Design review of the part built by this model. Coordinates are the model's own, in mm. A direction names the side the tool comes from. Give positions to 0.01 mm unless a question says otherwise; leave off trailing zeros. Loops run counter-clockwise (first coordinate to the right, second up) from the corner with the lowest first, then second, coordinate; pieces in that order, holes last. Notation, with made-up numbers: M 82.25,-33.75 L 111.25,-33.75 A16 ccw 111.25,-25.75 Z; hole C 23.5,44 d3. An arc over 180 degrees is marked long. Answer as CSV lines item,"result".
```python
from build123d import *

# Parameters (mm, degrees)
ESQUISSE1_W        = 5
ESQUISSE1_H        = 7
BOSS_EXTRU_1_DEPTH = 2.5
ESQUISSE2_R        = 0.25
BOSS_EXTRU_2_DEPTH = 23
ESQUISSE3_W        = 4
ESQUISSE3_H        = 6
BOSS_EXTRU_3_DEPTH = 2
CONG_1_R           = 2


with BuildPart() as part:
    # Esquisse1 → Boss.-Extru.1 (new body)
    with BuildSketch(Plane(origin=(0, 0, 0), x_dir=(1, 0, 0), z_dir=(0, 1, 0))):
        with Locations((2.5, 3.5)):
            Rectangle(ESQUISSE1_W, ESQUISSE1_H)
    extrude(amount=BOSS_EXTRU_1_DEPTH)

    # Esquisse2 → Boss.-Extru.2 (add)
    with BuildSketch(Plane.XY):
        with Locations(Location((0.5, 1.25, 0), (0, 0, 180))):
            Circle(ESQUISSE2_R)
        with Locations(Location((2.5, 1.25, 0), (0, 0, 180))):
            Circle(ESQUISSE2_R)
        with Locations(Location((4.5, 1.25, 0), (0, 0, 180))):
            Circle(ESQUISSE2_R)
    extrude(amount=BOSS_EXTRU_2_DEPTH)

    # Esquisse3 → Boss.-Extru.3 (add)
    with BuildSketch(Plane(origin=(0, 2.5, 0), x_dir=(1, 0, 0), z_dir=(0, 1, 0))):
        with Locations((2.5, 3)):
            Rectangle(ESQUISSE3_W, ESQUISSE3_H)
    extrude(amount=BOSS_EXTRU_3_DEPTH)

    # Congé1
    cong_1_edges = [part.edges().sort_by_distance(p)[0] for p in [
        (4.5, 4.5, -3),
        (2.5, 4.5, -6),
        (0.5, 4.5, -3),
    ]]
    fillet(cong_1_edges, radius=CONG_1_R - 0.0001)  # a hair under: the kernel refuses the full size


solid = part.part
```
1. For P1, Ø3, axis at x = 4.5, z = 10.5, coming from the -Y side; P2, Ø3, axis at x = 1, z = 13, coming from the +Y side, all flat-tipped, find the tip position at first contact; note any pin that passes through.
Answer block:
P1,"y = 1"
P2,"y = 1.5"
2. For faces 1 (the flat face through (2.3, 2.5, -6.4)), 2 (the flat face through (2, 0, -4)), list the 3-axis set-ups (+Z, -Z, +X, -X, +Y, -Y) from which the entire face can be reached by the end or side of a thin tool; tool diameter is ignored.
Answer block:
face 1,"-Z, +Y"
face 2,"+Z, -Z, +X, -X, -Y"
3. We need section B-B, the plane z = 14. Write out the cut boundary in (x, y).
Answer block:
outline,"C 0.5,1.25 d0.5; C 2.5,1.25 d0.5; C 4.5,1.25 d0.5"
4. We need section D-D, the plane y = 4.2. Write out the cut boundary in (x, z).
Answer block:
outline,"M 1.45,-5.05 L 3.55,-5.05 L 3.55,0 L 1.45,0 Z"
5. To check wall thickness, follow L1, parallel to X at y = 1.2, z = 10.75; L2, parallel to Z at x = 3, y = 2.15; L3, parallel to Z at x = 4.2, y = 2.6. State the ranges of each line that lie inside material, in increasing order. Write a range as [from, to].
Answer block:
L1,"[0.26, 0.74], [2.26, 2.74], [4.26, 4.74]"
L2,"[-7, 0]"
L3,"[-6, 0]"
6. The part is to be moulded in two halves that separate along Z. For faces 3 (the cylindrical face through (2.53, 3.63, -5.65)), 4 (the flat face through (2, 2, 0)), 5 (the flat face through (0, 1, -3)), say which applies: pulls with the +Z half, pulls with the -Z half, needs draft (parallel to the pull), parting line crosses it, or undercut.
Answer block:
face 3,"pulls with the -Z half"
face 4,"pulls with the +Z half"
face 5,"needs draft"
7. We need section A-A, the plane y = 1.25. Write out the cut boundary in (x, z), plus the area to 3 significant figures.
Answer block:
outline,"M 0,-7 L 5,-7 L 5,0 L 4.75,0 L 4.75,23 L 4.25,23 L 4.25,0 L 2.75,0 L 2.75,23 L 2.25,23 L 2.25,0 L 0.75,0 L 0.75,23 L 0.25,23 L 0.25,0 L 0,0 Z"
area,"69.5 mm²"
